Build history of the part. All positions in model axes, mm. A direction names the side the tool comes from. Give positions to 0.01 mm unless a question says otherwise; leave off trailing zeros. Order: outer loops, then holes, each group sorted by start corner. A loop starts at its lowest first (then second) coordinate and runs counter-clockwise, first axis right, second up. Notation, with made-up numbers: M 43.5,61 L 84.5,61 A16 ccw 84.5,91 Z; hole C -12,9 d10. An arc over 180 degrees is marked long. Answer as CSV lines item,"result".
from build123d import *

# Parameters (mm, degrees)
SCHIZZO1_W                   = 40
SCHIZZO1_H                   = 141
SCHIZZO1_R                   = 2.25
ESTRUSIONE_ESTRUSIONE4_DEPTH = 3
ESTRUSIONE_ESTRUSIONE5_DEPTH = 10
ESTRUSIONE_ESTRUSIONE6_DEPTH = 3.6
FORO_PER_VITE_M2_5_1_D       = 2.7


with BuildPart() as part:
    # Schizzo1 → Estrusione-Estrusione4 (new body)
    with BuildSketch(Plane.XY):
        Rectangle(SCHIZZO1_W, SCHIZZO1_H)
        with Locations((0, 44.5)):
            Circle(SCHIZZO1_R, mode=Mode.SUBTRACT)
        with Locations((0, -36.5)):
            Circle(SCHIZZO1_R, mode=Mode.SUBTRACT)
    extrude(amount=ESTRUSIONE_ESTRUSIONE4_DEPTH)

    # Schizzo2 → Estrusione-Estrusione5 (add)
    with BuildSketch(Plane.XY.offset(3)):
        with BuildLine():
            Line((15, 58), (15, 70.5))
            Line((15, 70.5), (12.5, 70.5))
            Line((12.5, 70.5), (12.5, 58))
            ThreePointArc((12.5, 58), (10.072584945, 50.597768409), (3.733114796, 46.070462963))
            ThreePointArc((3.733114796, 46.070462963), (4.03786402, 44.813295631), (3.930680514, 43.524166667))
            ThreePointArc((3.930680514, 43.524166667), (11.915540435, 48.888474544), (15, 58))
        make_face()
        with BuildLine():
            Line((-12.5, 58), (-12.5, 70.5))
            Line((-12.5, 70.5), (-15, 70.5))
            Line((-15, 70.5), (-15, 58))
            ThreePointArc((-15, 58), (-11.915540435, 48.888474544), (-3.930680514, 43.524166667))
            ThreePointArc((-3.930680514, 43.524166667), (-4.03786402, 44.813295631), (-3.733114796, 46.070462963))
            ThreePointArc((-3.733114796, 46.070462963), (-10.072584945, 50.597768409), (-12.5, 58))
        make_face()
    extrude(amount=ESTRUSIONE_ESTRUSIONE5_DEPTH)

    # Schizzo3 → Estrusione-Estrusione6 (add)
    with BuildSketch(Plane.XY.offset(3)):
        with BuildLine():
            Line((12.5, 58), (12.5, 70.5))
            Line((12.5, 70.5), (-12.5, 70.5))
            Line((-12.5, 70.5), (-12.5, 58))
            ThreePointArc((-12.5, 58), (-10.072584945, 50.597768409), (-3.733114796, 46.070462963))
            ThreePointArc((-3.733114796, 46.070462963), (0, 48.55), (3.733114796, 46.070462963))
            ThreePointArc((3.733114796, 46.070462963), (10.072584945, 50.597768409), (12.5, 58))
        make_face()
    extrude(amount=ESTRUSIONE_ESTRUSIONE6_DEPTH)

    # Foro per Vite M2.5-1 (through all)
    with Locations(Plane(origin=(-15, 33.524166667, 3), x_dir=(1, 0, 0), z_dir=(0, 0, 1))):
        with Locations((0, 0), (0, -94.024166667)):
            foro_per_vite_m2_5_1 = Hole(FORO_PER_VITE_M2_5_1_D / 2)

    # Specchia1: Foro per Vite M2.5-1 across plane
    add(foro_per_vite_m2_5_1.mirror(Plane(origin=(0, 0, 0), x_dir=(0, 0, 1), z_dir=(1, 0, 0))), mode=Mode.SUBTRACT)


solid = part.part
Item 1: 3-axis set-ups, long thin cutter, end or side, ignore diameter. For faces 1 (the flat face through (-12.5, 64, 10)), 2 (the cylindrical face through (12, 49, 8)), 3 (the cylindrical face through (-12, 49, 8)), 4 (the flat face through (0, 1, 0)): which of +Z, -Z, +X, -X, +Y, -Y reach the whole face in a straight line?
Geometry says:
face 1,"+Z, +Y"
face 2,"+Z, +X, -Y"
face 3,"+Z, -X, -Y"
face 4,"-Z, +X, -X, +Y, -Y"
Item 2: Band-saw the part on B-B (y = -60.5). Give the cut face in (x, z), and give its area (3 significant figures).
Geometry says:
outline,"M -20,0 L -16.35,0 L -16.35,3 L -20,3 Z; M -13.65,0 L 13.65,0 L 13.65,3 L -13.65,3 Z; M 16.35,0 L 20,0 L 20,3 L 16.35,3 Z"
area,"104 mm2"
Item 3: Drop flat-ended pins along their axis: pin 1 (3 mm diameter, centred on y = 61.5, z = 8.5, fed in from -X); pin 2 (12 mm diameter, centred on x = 8.5, y = 19, fed in from +Z); pin 3 (12 mm diameter, centred on x = -6, y = 62, fed in from +Z). Give the stop position or say it passes through.
Geometry says:
pin 1,"stops at x = -15"
pin 2,"stops at z = 3"
pin 3,"stops at z = 6.6"
Item 4: Pull direction Y, two halves, no side cores. Call faces 5 (the flat face through (13, 55, 13)), 6 (the flat face through (0, -70.5, 1)), 7 (the cylindrical face through (-14.824, 34.863, 1.479)), 8 (the cylindrical face through (-14.71, -61.82, 1.48)): released by +Y, released by -Y, zero draft, split by the parting line, or undercut.
Geometry says:
face 5,"zero draft"
face 6,"released by -Y"
face 7,"undercut"
face 8,"undercut"
Item 5: Band-saw the part on A-A (x = 0). Give the cut face in (y, z), and give its area (3 significant figures).
Geometry says:
outline,"M -70.5,0 L -38.75,0 L -38.75,3 L -70.5,3 Z; M -34.25,0 L 42.25,0 L 42.25,3 L -34.25,3 Z; M 46.75,0 L 70.5,0 L 70.5,6.6 L 48.55,6.6 L 48.55,3 L 46.75,3 Z"
area,"475 mm2"
Item 6: Band-saw the part on C-C (z = 11). Give the cut face in (x, y), and give its area (3 significant figures).
Geometry says:
outline,"M -15,58 A15 ccw -3.93,43.52 A4.05 cw -3.73,46.07 A12.5 cw -12.5,58 L -12.5,70.5 L -15,70.5 Z; M 3.73,46.07 A4.05 cw 3.93,43.52 A15 ccw 15,58 L 15,70.5 L 12.5,70.5 L 12.5,58 A12.5 cw Z"
area,"150 mm2"
Item 7: Band-saw the part on D-D (x = 10.5). Give the cut face in (y, z), and give its area (3 significant figures).
Geometry says:
outline,"M -70.5,0 L 70.5,0 L 70.5,6.6 L 51.22,6.6 L 51.22,13 L 47.29,13 L 47.29,3 L -70.5,3 Z"
area,"532 mm2"
Item 8: Probe line 1 along Y through (x, z) = (-15, 0.85); line 2 along Y through (x, z) = (0, 1.65); line 3 along Z through (x, y) = (-5.5, -20.5). List the from-to ranges inside material, lowest first. Write a range as from..to.
Geometry says:
line 1,"y = -70.5..-61.85, -59.15..32.17, 34.87..70.5"
line 2,"y = -70.5..-38.75, -34.25..42.25, 46.75..70.5"
line 3,"z = 0..3"
